Can you work these out from the model? Positions are in its coordinate system, mm. Coordinates: 2 decimals unless noted, no trailing zeros. Order: outer loops, then holes, each group sorted by start corner. A loop starts at its lowest first (then second) coordinate and runs counter-clockwise, first axis right, second up. Notation, with made-up numbers: (19.5, 15) - (76.5, 15) arc R7 cw to (76.5, 27) - close; hole circle Ø1 at (61, 63). An arc over 180 degrees is marked (long way). Return JSON: item names as keys, results as strings. Group by question number.
1) Imagine slicing it at B-B (z = 0.75). Give the number of separate pieces and of enclosed holes in the cut face, and give its area (3 significant figures).
2) If we mould it in two halves opening along X, with no side actions, what happens to faces 1 (the face through (25, -88, 0.5)), 2 (the face through (-39.735, -92.218, 0.493)), 3 (the face through (-48.61, -77.99, 0.49))? For each: pulls with the +X half, pulls with the -X half, needs draft (parallel to the pull), parting line crosses it, or undercut.
3) For pin 1 Ø2.5 at (x, y) = (-47.5, 71) entering from -Z, with a flat end and sliding along its axis, tell me the tip position at first contact or that it passes through.
4) Imagine slicing it at A-A (y = 51.5). Write out the boundary of the cut face in (x, z).
5) If I drill on line 1 along X through (y, z) = (-79, 0.35); line 2 along X through (y, z) = (-7.5, 0.9); line 3 along Y through (x, z) = (27.5, 0.45), over which ranges is the centre line in solid material (lowest first)?
```python
from build123d import *

# Parameters (mm, degrees)
SKETCH2_R           = 1.5
BOSS_EXTRUDE1_DEPTH = 1


with BuildPart() as part:
    # Sketch2 → Boss-Extrude1 (new body)
    with BuildSketch(Plane.XY):
        with BuildLine():
            Line((-35.857864376, -93), (15.857864376, -93))
            ThreePointArc((15.857864376, -93), (19.6846987, -92.238795325), (22.928932188, -90.071067812))
            Line((22.928932188, -90.071067812), (27.071067812, -85.928932188))
            ThreePointArc((27.071067812, -85.928932188), (29.238795325, -82.6846987), (30, -78.857864376))
            Line((30, -78.857864376), (30, 71))
            ThreePointArc((30, 71), (29.121320344, 73.121320344), (27, 74))
            Line((27, 74), (-47, 74))
            ThreePointArc((-47, 74), (-49.121320344, 73.121320344), (-50, 71))
            Line((-50, 71), (-50, -78.857864376))
            ThreePointArc((-50, -78.857864376), (-49.238795325, -82.6846987), (-47.071067812, -85.928932188))
            Line((-47.071067812, -85.928932188), (-42.928932188, -90.071067812))
            ThreePointArc((-42.928932188, -90.071067812), (-39.6846987, -92.238795325), (-35.857864376, -93))
        make_face()
        with Locations((-47.5, 71)):
            Circle(SKETCH2_R, mode=Mode.SUBTRACT)
        with Locations((27.5, 71)):
            Circle(SKETCH2_R, mode=Mode.SUBTRACT)
        with Locations((-47.5, -79)):
            Circle(SKETCH2_R, mode=Mode.SUBTRACT)
        with Locations((27.5, -79)):
            Circle(SKETCH2_R, mode=Mode.SUBTRACT)
        with BuildLine():
            Line((-48.5, -12), (-48.5, 4))
            ThreePointArc((-48.5, 4), (-47, 5.5), (-45.5, 4))
            Line((-45.5, 4), (-45.5, -12))
            ThreePointArc((-45.5, -12), (-47, -13.5), (-48.5, -12))
        make_face(mode=Mode.SUBTRACT)
        with BuildLine():
            Line((28.5, -12), (28.5, 4))
            ThreePointArc((28.5, 4), (27, 5.5), (25.5, 4))
            Line((25.5, 4), (25.5, -12))
            ThreePointArc((25.5, -12), (27, -13.5), (28.5, -12))
        make_face(mode=Mode.SUBTRACT)
        with BuildLine():
            Line((-48.5, 38), (-48.5, 54))
            ThreePointArc((-48.5, 54), (-47, 55.5), (-45.5, 54))
            Line((-45.5, 54), (-45.5, 38))
            ThreePointArc((-45.5, 38), (-47, 36.5), (-48.5, 38))
        make_face(mode=Mode.SUBTRACT)
        with BuildLine():
            Line((-45.5, -46), (-45.5, -62))
            ThreePointArc((-45.5, -62), (-47, -63.5), (-48.5, -62))
            Line((-48.5, -62), (-48.5, -46))
            ThreePointArc((-48.5, -46), (-47, -44.5), (-45.5, -46))
        make_face(mode=Mode.SUBTRACT)
        with BuildLine():
            Line((28.5, 38), (28.5, 54))
            ThreePointArc((28.5, 54), (27, 55.5), (25.5, 54))
            Line((25.5, 54), (25.5, 38))
            ThreePointArc((25.5, 38), (27, 36.5), (28.5, 38))
        make_face(mode=Mode.SUBTRACT)
        with BuildLine():
            Line((25.5, -46), (25.5, -62))
            ThreePointArc((25.5, -62), (27, -63.5), (28.5, -62))
            Line((28.5, -62), (28.5, -46))
            ThreePointArc((28.5, -46), (27, -44.5), (25.5, -46))
        make_face(mode=Mode.SUBTRACT)
    extrude(amount=BOSS_EXTRUDE1_DEPTH)


solid = part.part
```
Calculated:
{
 "1": {"separate pieces": "1", "enclosed holes": "10", "area": "12,900 mm2"},
 "2": {"face 1": "pulls with the +X half", "face 2": "pulls with the -X half", "face 3": "undercut"},
 "3": {"pin 1": "through"},
 "4": {"outline": "(-50, 0) - (-48.5, 0) - (-48.5, 1) - (-50, 1) - close; (-45.5, 0) - (25.5, 0) - (25.5, 1) - (-45.5, 1) - close; (28.5, 0) - (30, 0) - (30, 1) - (28.5, 1) - close"},
 "5": {"line 1": "-50 to -49, -46 to 26, 29 to 30", "line 2": "-50 to -48.5, -45.5 to 25.5, 28.5 to 30", "line 3": "-85.47 to -80.5, -77.5 to -63.41, -44.59 to -13.41, 5.41 to 36.59, 55.41 to 69.5, 72.5 to 73.96"}
}
